Design review of the part built by this model. Coordinates are the model's own, in mm. Face numbers are marked on the shaded views. Give positions to 0.01 mm unless a question says otherwise; leave off trailing zeros. Order: outer loops, then holes, each group sorted by start corner. A loop starts at its lowest first (then second) coordinate and runs counter-clockwise, first axis right, second up. Notation, with made-up numbers: (54, 69.25) -> (65, 69.25) arc R13 ccw to (65, 80.25) -> close; hole circle Ø10 at (42, 43). An arc over 180 degrees is marked (long way). One line per item, written item: value. Start each with the question number.
1) Consider section A-A (y = 42). State the section outline as (x, z) points (3 decimals).
2) The part is to be moulded in two halves that separate along X. For the marked faces 1, 2, 3 and 4, say which applies: released by +X, released by -X, zero draft, split by the parting line, or undercut.
3) Wall thickness on line 1 along Y through (x, z) = (14.25, 2.95); line 2 along Y through (x, z) = (18.5, 0.75); line 3 along X through (y, z) = (37, 2.25): over which ranges is each line inside the solid? List them lowest first. Write a range as from..to.
4) Consider section D-D (y = 4). State the section outline as (x, z) points (3 decimals), plus the area to 3 significant figures.
5) Consider section C-C (z = 0.75). State the section outline as (x, y) points (3 decimals), plus the area to 3 significant figures.
6) Consider section B-B (x = 8.75). State the section outline as (y, z) points (3 decimals), plus the area to 3 significant figures.
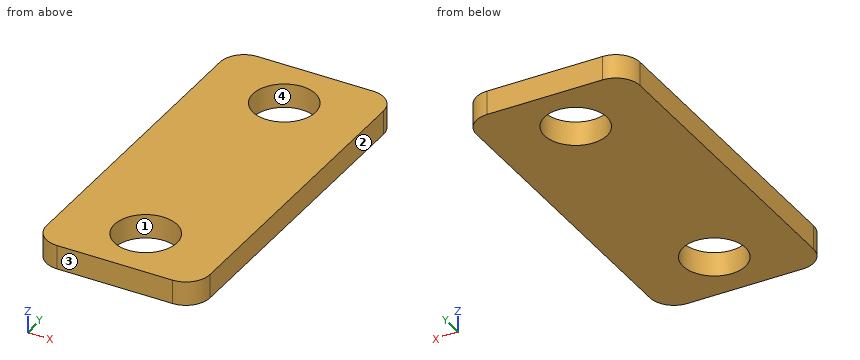
from build123d import *

# Parameters (mm, degrees)
SKETCH1_W           = 21.59
SKETCH1_H           = 46.99
SKETCH1_R           = 4.124999878
BOSS_EXTRUDE1_DEPTH = 3.175
FILLET1_R           = 3.175


with BuildPart() as part:
    # Sketch1 → Boss-Extrude1 (new body)
    with BuildSketch(Plane.XY):
        with Locations((10.795, 23.495)):
            Rectangle(SKETCH1_W, SKETCH1_H)
        with Locations((10.795, 7.260198401)):
            Circle(SKETCH1_R, mode=Mode.SUBTRACT)
        with Locations(Location((10.795, 39.729801599, 0), (0, 0, 180))):
            Circle(SKETCH1_R, mode=Mode.SUBTRACT)
    extrude(amount=BOSS_EXTRUDE1_DEPTH)

    # Fillet1
    fillet1_edges = [part.edges().sort_by_distance(p)[0] for p in [
        (0, 0, 1.5875),
        (21.59, 0, 1.5875),
        (21.59, 46.99, 1.5875),
        (0, 46.99, 1.5875),
    ]]
    fillet(fillet1_edges, radius=FILLET1_R)


solid = part.part
Checked values:
1. outline: (0, 0) -> (7.351, 0) -> (7.351, 3.175) -> (0, 3.175) -> close; (14.239, 0) -> (21.59, 0) -> (21.59, 3.175) -> (14.239, 3.175) -> close
2. face 1: undercut
2. face 2: released by +X
2. face 3: zero draft
2. face 4: undercut
3. line 1: y = 0..5.01, 9.51..37.48, 41.98..46.99
3. line 2: y = 0..46.99
3. line 3: x = 0..7.7, 13.89..21.59
4. outline: (0, 0) -> (8.268, 0) -> (8.268, 3.175) -> (0, 3.175) -> close; (13.322, 0) -> (21.59, 0) -> (21.59, 3.175) -> (13.322, 3.175) -> close
4. area: 52.5 mm^2
5. outline: (0, 3.175) arc R3.175 ccw to (3.175, 0) -> (18.415, 0) arc R3.175 ccw to (21.59, 3.175) -> (21.59, 43.815) arc R3.175 ccw to (18.415, 46.99) -> (3.175, 46.99) arc R3.175 ccw to (0, 43.815) -> close; hole circle Ø8.25 at (10.795, 7.26); hole circle Ø8.25 at (10.795, 39.73)
5. area: 899 mm^2
6. outline: (0, 0) -> (3.678, 0) -> (3.678, 3.175) -> (0, 3.175) -> close; (10.843, 0) -> (36.147, 0) -> (36.147, 3.175) -> (10.843, 3.175) -> close; (43.312, 0) -> (46.99, 0) -> (46.99, 3.175) -> (43.312, 3.175) -> close
6. area: 104 mm^2
